For this review, take the finished solid that the model builds, in its own axes (mm). Face numbers are marked on the shaded views. Give positions to 0.01 mm unless a question says otherwise; leave off trailing zeros. Write each loop counter-clockwise with the first axis right and the second up, starting at its lowest first coordinate (ties: lowest second). Pieces come first, ordered by that corner, then holes.
Q1. Insertion check: P1, Ø0.9, axis at x = 37, y = 37, coming from the +Z side. The pin has a flat end and moves straight along its axis. Give the tip position at first contact, or say it passes through.
Q2. We need section A-A (z = 8). Write out the cut boundary in (x, y).
Q3. Mouldability with a two-part tool opening along Y and no side actions: class the marked faces 1, 2 and 3 as released by +Y, released by -Y, zero draft, split by the parting line, or undercut.
Q4. We need section B-B (y = 37). Write out the cut boundary in (x, z).
Q5. For line 1 (Y direction, x = 37, z = 6.5); line 2 (X direction, y = 35.5, z = 4.5), list the stretches that pass through material, from the lowest coordinate up.
```python
from build123d import *

# Parameters (mm, degrees)
SKETCH1_W             = 40
SKETCH1_H             = 40
BOSS_EXTRUDE1_DEPTH   = 10
F_3_0MM_DOWEL_HOLE1_D = 1.524
MIRROR2_COPY_1_D      = 1.524
FILLET1_R             = 5


with BuildPart() as part:
    # Sketch1 → Boss-Extrude1 (new body)
    with BuildSketch(Plane.XY):
        with Locations((20, 20)):
            Rectangle(SKETCH1_W, SKETCH1_H)
    extrude(amount=BOSS_EXTRUDE1_DEPTH)

    # Ø3.0mm Dowel Hole1 (through all)
    with Locations(Plane.XY.offset(10)):
        with Locations((3, 37)):
            f_3_0mm_dowel_hole1 = Hole(F_3_0MM_DOWEL_HOLE1_D / 2)

    # Mirror1: Ø3.0mm Dowel Hole1 across plane
    add(f_3_0mm_dowel_hole1.mirror(Plane.ZY.offset(-20)), mode=Mode.SUBTRACT)

    # Mirror2: Ø3.0mm Dowel Hole1 across plane
    add(f_3_0mm_dowel_hole1.mirror(Plane.ZX.offset(20)), mode=Mode.SUBTRACT)

    # Mirror2 copy 1 (through all)
    with Locations(Plane(origin=(40, 40, 10), x_dir=(-1, 0, 0), z_dir=(0, 0, 1))):
        with Locations((3, 37)):
            Hole(MIRROR2_COPY_1_D / 2)

    # Fillet1
    fillet1_edges = [part.edges().sort_by_distance(p)[0] for p in [
        (0, 40, 5),
        (40, 40, 5),
        (40, 0, 5),
        (0, 0, 5),
    ]]
    fillet(fillet1_edges, radius=FILLET1_R)


solid = part.part
```
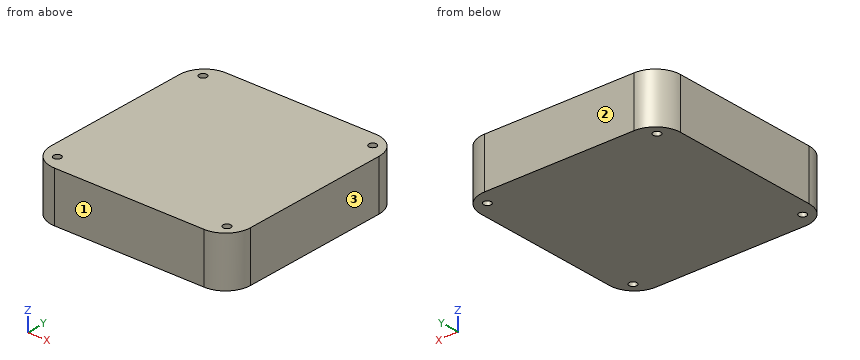
Computed:
1. P1: passes through
2. outline: (0, 5) arc R5 ccw to (5, 0) - (35, 0) arc R5 ccw to (40, 5) - (40, 35) arc R5 ccw to (35, 40) - (5, 40) arc R5 ccw to (0, 35) - close; hole circle Ø1.52 at (3, 3); hole circle Ø1.52 at (3, 37); hole circle Ø1.52 at (37, 3); hole circle Ø1.52 at (37, 37)
3. face 1: released by -Y
3. face 2: released by +Y
3. face 3: zero draft
4. outline: (0.42, 0) - (2.24, 0) - (2.24, 10) - (0.42, 10) - close; (3.76, 0) - (36.24, 0) - (36.24, 10) - (3.76, 10) - close; (37.76, 0) - (39.58, 0) - (39.58, 10) - (37.76, 10) - close
5. line 1: y = 0.42 to 2.24, 3.76 to 36.24, 37.76 to 39.58
5. line 2: x = 0.03 to 39.97
